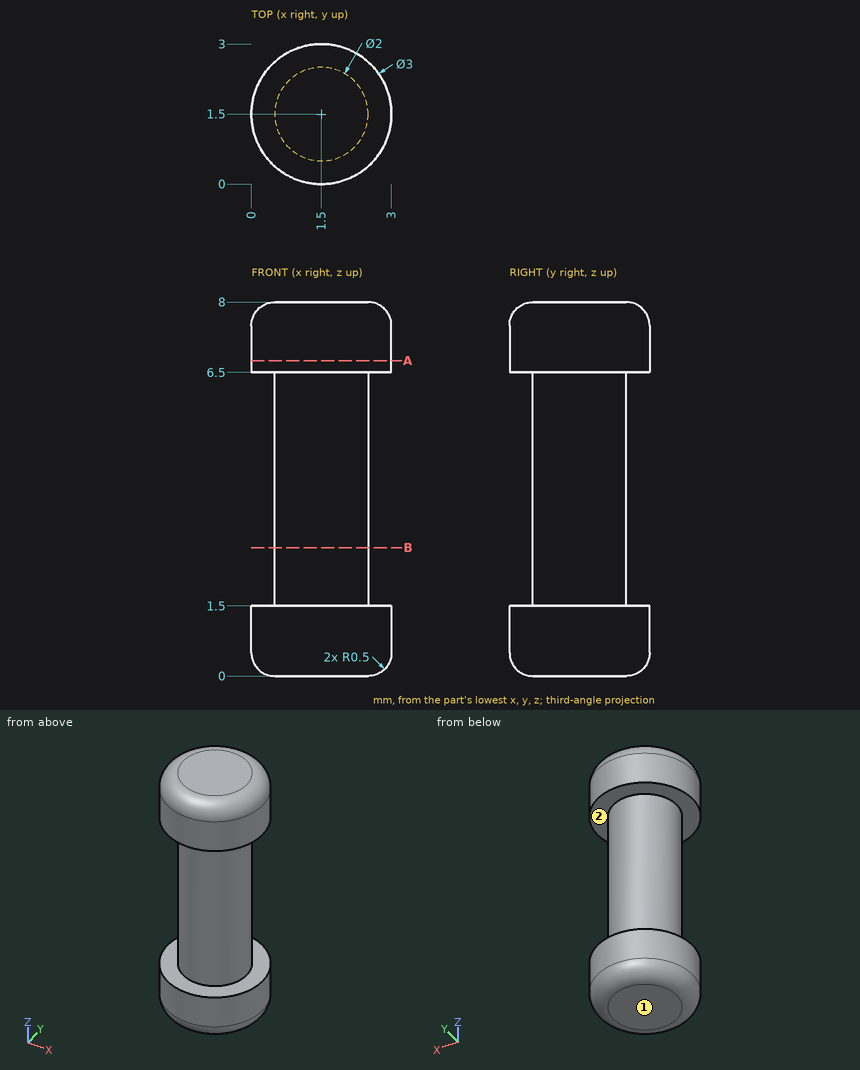
Verification items for this drawing (mm, ordinates from the low corner). A direction names the side the tool comes from. Coordinates: 2 decimals unless noted, no trailing zeros. Order: outer loops, then holes, each group sorted by start corner. A loop starts at its lowest first (then second) coordinate and runs counter-clockwise, first axis right, second up. Notation, with made-up numbers: (11.25, 3.5) -> (62.25, 3.5) arc R21 ccw to (62.25, 7.5) -> close; hole circle Ø8 at (-15, 20). An arc over 180 degrees is marked (long way). Put each result on its own line as item: value. Start each with the question number.
1. Cross-section at A-A, the plane z = 6.75. Record the boundary of the cut face in (x, y), then the cut area to 3 significant figures.
2. Material ranges on L1, parallel to Z at x = 0.6, y = 1; L2, parallel to Z at x = 2.35, y = 0.55; L3, parallel to X at y = 1.55, z = 3.5, recorded low to high. Write a range as [from, to].
3. Cross-section at B-B, the plane z = 2.75. Record the boundary of the cut face in (x, y).
4. Go/stop test with a flat-tipped pin: pin 1 Ø1.5 at (x, z) = (1.5, 2.5) entering from -Y. Record where the tip stops, or that it passes through.
5. Access from +Z, -Z, +X, -X, +Y, -Y to the whole of each face (thin tool, end or side, straight path). Record for the marked faces 1 and 2.
Computed:
1. outline: circle Ø3 at (1.5, 1.5)
1. area: 7.07 mm2
2. L1: [0, 1.5], [6.5, 8]
2. L2: [0.08, 1.5], [6.5, 7.92]
2. L3: [0.5, 2.5]
3. outline: circle Ø2 at (1.5, 1.5)
4. pin 1: y = 0.5
5. face 1: -Z, +X, -X, +Y, -Y
5. face 2: none
